The listing builds one solid part. Answer for the finished solid, in the listing's coordinates (mm). Face numbers are marked on the shaded views. A direction names the side the tool comes from. Round coordinates to 2 decimals unless told otherwise and drop trailing zeros. Loops run counter-clockwise (first coordinate to the right, second up) from the corner with the lowest first, then second, coordinate; pieces in that order, holes last. Notation, with made-up numbers: M -39,-12.5 L -4,-12.5 A31 cw -4,19.5 Z; hole C 26.5,10.25 d4. An arc over 180 degrees is marked long. Put each result on its own line as item: value. Start each with the question number.
(1) Section A-A, the plane y = 36 is taken. Determine the outline of the cut face in (x, z) (3 decimals), then the cut area to 3 significant figures.
(2) Which of the six approach directions +Z, -Z, +X, -X, +Y, -Y give full straight-line access (tool end or side, diameter ignored) to the marked faces 1 and 2?
(3) Section C-C, the plane z = -11 is taken. Determine the outline of the cut face in (x, y) (3 decimals).
(4) Section B-B, the plane x = 8.5 is taken. Determine the outline of the cut face in (y, z) (3 decimals).
(5) Flat-ended cylindrical pins translate along their axes: P1, Ø5.5, axis at x = 13.5, y = 51, coming from the -Z side (3 decimals); P2, Ø2, axis at y = 76, z = -15, coming from the +X side (3 decimals). Find the tip coordinate at first contact, or state that the pin passes through.
(6) Straight lines are drawn through the part: line 1 (X direction, y = 71.5, z = -10) (3 decimals); line 2 (Z direction, x = 16, y = 52.5) (3 decimals); line 3 (X direction, y = 37, z = -4.25). For each, find the intervals that lie inside material, in ascending order.
```python
from build123d import *

# Parameters (mm, degrees)
BOSS_EXTRUDE1_DEPTH = 123.952
FILLET1_R           = 2.54


with BuildPart() as part:
    # Sketch1 → Boss-Extrude1 (new body)
    with BuildSketch(Plane(origin=(0, 0, 0), x_dir=(1, 0, 0), z_dir=(0, 1, 0))):
        Polygon((0, 0), (0, 19.05), (3.175, 19.05), (3.175, 3.175), (19.05, 3.175), (19.05, 0), align=None)
    extrude(amount=BOSS_EXTRUDE1_DEPTH)

    # Fillet1
    fillet1_edges = [part.edges().sort_by_distance(p)[0] for p in [
        (3.175, 61.976, -19.05),
        (3.175, 61.976, -3.175),
        (19.05, 61.976, -3.175),
    ]]
    fillet(fillet1_edges, radius=FILLET1_R)


solid = part.part
```
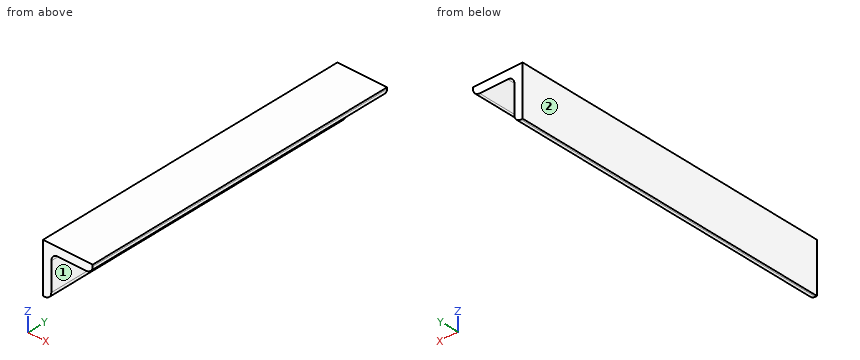
Recorded:
1. outline: M 0,-19.05 L 0.635,-19.05 A2.54 ccw 3.175,-16.51 L 3.175,-5.715 A2.54 cw 5.715,-3.175 L 16.51,-3.175 A2.54 ccw 19.05,-0.635 L 19.05,0 L 0,0 Z
1. area: 110 mm²
2. face 1: -Z, +X, +Y, -Y
2. face 2: +Z, -Z, -X, +Y, -Y
3. outline: M 0,0 L 3.175,0 L 3.175,123.952 L 0,123.952 Z
4. outline: M 0,-3.175 L 123.952,-3.175 L 123.952,0 L 0,0 Z
5. P1: stops at z = -3.175
5. P2: stops at x = 3.175
6. line 1: x = 0 to 3.175
6. line 2: z = -3.175 to 0
6. line 3: x = 0 to 3.64
